Check sheet for the modelled part. Datum: model origin and axes. Units: mm. A direction names the side the tool comes from. Round coordinates to 2 decimals unless told otherwise and drop trailing zeros. Write each loop counter-clockwise with the first axis right and the second up, starting at its lowest first coordinate (ties: lowest second). Pieces come first, ordered by that corner, then holes.
Item 1: Go/stop test with flat-tipped pins: pin 1 Ø9 at (y, z) = (12, -10) entering from +X; pin 2 Ø2.5 at (y, z) = (12, -8) entering from -X; pin 3 Ø8 at (y, z) = (7, -1) entering from +X; pin 4 Ø6 at (x, z) = (32, -8) entering from +Y. Record where each tip stops, or that it passes through.
Item 2: Cross-section at A-A on x = 22. Enter the section's corners in (y, z).
Item 3: Cross-section at C-C on y = 12.75. Enter the section's corners in (x, z), plus the area to 3 significant figures.
Item 4: Release check for a two-part mould opening along X. For faces 4 (the cylindrical face through (26.16, 11.06, -15.62)), 5 (the cylindrical face through (-23.91, 4.4, 3.24)), 6 (the flat face through (-7.949, 3.944, -3.495)), 7 (the flat face through (-13.5, 8, -8.2)) record: +X half, -X half, draft (parallel to the pull), parting line (faces both ways), or undercut.
Item 5: Cross-section at D-D on x = -7. Enter the section's corners in (y, z).
Item 6: Cross-section at B-B on z = -12.75. Enter the section's corners in (x, y), plus the area to 3 significant figures.
Item 7: Material ranges on line 1 (Z direction, x = -11.5, y = 12.75); line 2 (X direction, y = 1.5, z = -9.75); line 3 (X direction, y = 4.75, z = -7.25), recorded low to high.
Item 8: Tool access check on faces 1 (the cylindrical face through (24.35, 11.55, -5.12)), 2 (the flat face through (17.786, 3.944, -7.689)), 3 (the cylindrical face through (-23.907, 4.399, -15.617)). Record the directions out of +Z, -Z, +X, -X, +Y, -Y that give a thin tool (end or side, any length) a straight path to the whole face; none if there is none.
from build123d import *

# Parameters (mm, degrees)
SKETCH1_W           = 70
SKETCH1_H           = 20
BOSS_EXTRUDE1_DEPTH = 5
SKETCH2_W           = 43
SKETCH2_H           = 20
BOSS_EXTRUDE2_DEPTH = 10
FILLET1_R           = 2
SKETCH3_R           = 2.8
CUT_EXTRUDE1_DEPTH  = 16
CUT_EXTRUDE2_DEPTH  = 8


with BuildPart() as part:
    # Sketch1 → Boss-Extrude1 (new body)
    with BuildSketch(Plane(origin=(0, 0, 0), x_dir=(1, 0, 0), z_dir=(0, 1, 0))):
        with Locations((5.262356584, 6.187481613)):
            Rectangle(SKETCH1_W, SKETCH1_H)
    extrude(amount=BOSS_EXTRUDE1_DEPTH)

    # Sketch2 → Boss-Extrude2 (add)
    with BuildSketch(Plane(origin=(0, 5, 0), x_dir=(1, 0, 0), z_dir=(0, 1, 0))):
        with Locations((5.262356584, 6.187481613)):
            Rectangle(SKETCH2_W, SKETCH2_H)
    extrude(amount=BOSS_EXTRUDE2_DEPTH)

    # Fillet1
    fillet1_edges = [part.edges().sort_by_distance(p)[0] for p in [
        (-22.987643416, 5, 3.812518387),
        (-22.987643416, 5, -16.187481613),
        (33.512356584, 5, 3.812518387),
        (26.762356584, 5, -6.187481613),
        (26.762356584, 10, 3.812518387),
        (26.762356584, 10, -16.187481613),
        (-16.237643416, 5, -6.187481613),
        (-16.237643416, 10, -16.187481613),
        (-16.237643416, 10, 3.812518387),
        (33.512356584, 5, -16.187481613),
    ]]
    fillet(fillet1_edges, radius=FILLET1_R)

    # Sketch3 → Cut-Extrude1 (cut, through all)
    with BuildSketch(Plane(origin=(0, 15, 0), x_dir=(1, 0, 0), z_dir=(0, 1, 0))):
        with Locations((21.762356584, 6.187481613)):
            Circle(SKETCH3_R)
        with Locations((-11.237643416, 6.187481613)):
            Circle(SKETCH3_R)
    extrude(amount=-CUT_EXTRUDE1_DEPTH, mode=Mode.SUBTRACT)

    # Sketch4 → Cut-Extrude2 (cut)
    with BuildSketch(Plane.XZ):
        Polygon((-8.098072068, -9.959274965), (-6.401388882, -5.354429745), (-9.54096023, -1.582636394), (-14.377214764, -2.415688262), (-16.07389795, -7.020533482), (-12.934326602, -10.792326833), align=None)
        Polygon((23.45903977, -10.792326833), (18.622785236, -9.959274965), (16.92610205, -5.354429745), (20.065673398, -1.582636394), (24.901927932, -2.415688262), (26.598611118, -7.020533482), align=None)
    extrude(amount=-CUT_EXTRUDE2_DEPTH, mode=Mode.SUBTRACT)


solid = part.part
Response values:
1. pin 1: stops at x = 26.76
1. pin 2: stops at x = -16.24
1. pin 3: stops at x = 40.26
1. pin 4: stops at y = 5
2. outline: (0, -16.19) - (15, -16.19) - (15, -8.98) - (8, -8.98) - (8, -10.54) - (0, -10.54) - close; (0, -1.92) - (8, -1.92) - (8, -3.4) - (15, -3.4) - (15, 3.81) - (0, 3.81) - close
3. outline: (-16.24, -14.19) arc R2 ccw to (-14.24, -16.19) - (24.76, -16.19) arc R2 ccw to (26.76, -14.19) - (26.76, 1.81) arc R2 ccw to (24.76, 3.81) - (-14.24, 3.81) arc R2 ccw to (-16.24, 1.81) - close; hole circle Ø5.6 at (-11.24, -6.19); hole circle Ø5.6 at (21.76, -6.19)
3. area: 807 mm2
4. face 4: +X half
4. face 5: draft
4. face 6: undercut
4. face 7: undercut
5. outline: (0, -16.19) - (15, -16.19) - (15, 3.81) - (0, 3.81) - (0, -4.64) - (8, -4.64) - (8, -6.98) - (0, -6.98) - close
6. outline: (-29.74, 0) - (40.26, 0) - (40.26, 5) - (28.76, 5) arc R2 cw to (26.76, 7) - (26.76, 15) - (-16.24, 15) - (-16.24, 7) arc R2 cw to (-18.24, 5) - (-29.74, 5) - close
6. area: 782 mm2
7. line 1: z = -16.19 to -8.98, -3.4 to 3.81
7. line 2: x = -29.74 to -13.8, -8.02 to 18.55, 24.33 to 40.26
7. line 3: x = -29.74 to -15.88, -7.1 to 17.62, 26.41 to 40.26
8. face 1: +Y, -Y
8. face 2: -Y
8. face 3: -Z, -X, +Y
